```python
from build123d import *

# Parameters (mm, degrees)
FACE005_W        = 5
FACE005_H        = 52
EXTRUDE005_DEPTH = 1.6
FACE004_R        = 5
EXTRUDE004_DEPTH = 1.5
EXTRUDE003_DEPTH = 2
FACE002_R        = 1.25
EXTRUDE002_DEPTH = 10
FACE001_R        = 2.5
EXTRUDE001_DEPTH = 10
EXTRUDE_DEPTH    = 6.5


with BuildPart() as extrude005:
    # Face005 → Extrude005 (new body)
    with BuildSketch(Plane(origin=(34, 28, 5), x_dir=(0, 1, 0), z_dir=(0, 0, 1))):
        Rectangle(FACE005_W, FACE005_H)
    extrude(amount=-EXTRUDE005_DEPTH)


with BuildPart() as extrude004:
    # Face004 → Extrude004 (new body)
    with BuildSketch(Plane(origin=(34, 16.5, 6.5), x_dir=(0, 1, 0), z_dir=(0, 0, 1))):
        with BuildLine():
            ThreePointArc((15.5, 29), (14.328427, 31.828427), (11.5, 33))
            Line((11.5, 33), (-11.5, 33))
            ThreePointArc((-11.5, 33), (-14.328427, 31.828427), (-15.5, 29))
            Line((-15.5, 29), (-15.5, -29))
            ThreePointArc((-15.5, -29), (-14.328427, -31.828427), (-11.5, -33))
            Line((-11.5, -33), (11.5, -33))
            ThreePointArc((11.5, -33), (14.328427, -31.828427), (15.5, -29))
            Line((15.5, -29), (15.5, 29))
        make_face()
        with Locations((24.5, 26)):
            Circle(FACE004_R)
        with Locations((24.5, -26)):
            Circle(FACE004_R)
    extrude(amount=-EXTRUDE004_DEPTH)


with BuildPart() as extrude003:
    # Face003 → Extrude003 (new body)
    with BuildSketch(Plane(origin=(5, 5, 0), x_dir=(0, 1, 0), z_dir=(0, 0, 1))):
        Polygon((-1.443376, -2.5), (1.443376, -2.5), (2.886751, 0), (1.443376, 2.5), (-1.443376, 2.5), (-2.886751, 0), align=None)
        Polygon((24.443376, -60.5), (25.886751, -58), (24.443376, -55.5), (21.556624, -55.5), (20.113249, -58), (21.556624, -60.5), align=None)
        Polygon((1.443376, -60.5), (2.886751, -58), (1.443376, -55.5), (-1.443376, -55.5), (-2.886751, -58), (-1.443376, -60.5), align=None)
        Polygon((24.443376, -2.5), (25.886751, 0), (24.443376, 2.5), (21.556624, 2.5), (20.113249, 0), (21.556624, -2.5), align=None)
    extrude(amount=EXTRUDE003_DEPTH)


with BuildPart() as extrude002:
    # Face002 → Extrude002 (new body)
    with BuildSketch(Plane(origin=(63, 28, 6.5), x_dir=(0, 1, 0), z_dir=(0, 0, 1))):
        Circle(FACE002_R)
        with Locations((-23, 0)):
            Circle(FACE002_R)
        with Locations((-23, 58)):
            Circle(FACE002_R)
        with Locations((0, 58)):
            Circle(FACE002_R)
    extrude(amount=-EXTRUDE002_DEPTH)


with BuildPart() as extrude001:
    # Face001 → Extrude001 (new body)
    with BuildSketch(Plane(origin=(60, 41, 6.5), x_dir=(0, 1, 0), z_dir=(0, 0, 1))):
        Circle(FACE001_R)
        with Locations((0, 52)):
            Circle(FACE001_R)
    extrude(amount=-EXTRUDE001_DEPTH)


with BuildPart() as cut004:
    # Face → Extrude (new body)
    with BuildSketch(Plane(origin=(34, 24.5, 0), x_dir=(0, 1, 0), z_dir=(0, 0, 1))):
        with BuildLine():
            ThreePointArc((-19.5, 34), (-23.035534, 32.535534), (-24.5, 29))
            Line((-24.5, 29), (-24.5, -29.000001))
            ThreePointArc((-24.5, -29.000001), (-23.035534, -32.535534), (-19.5, -34))
            Line((-19.5, -34), (19.5, -34))
            ThreePointArc((19.5, -34), (23.035534, -32.535534), (24.5, -29))
            Line((24.5, -29), (24.5, 29))
            ThreePointArc((24.5, 29), (23.035534, 32.535534), (19.5, 34))
            Line((19.5, 34), (-19.5, 34))
        make_face()
    extrude(amount=EXTRUDE_DEPTH)

    # Cut: cut Extrude001
    add(extrude001.part, mode=Mode.SUBTRACT)

    # Cut001: cut Extrude002
    add(extrude002.part, mode=Mode.SUBTRACT)

    # Cut002: cut Extrude003
    add(extrude003.part, mode=Mode.SUBTRACT)

    # Cut003: cut Extrude004
    add(extrude004.part, mode=Mode.SUBTRACT)

    # Cut004: cut Extrude005
    add(extrude005.part, mode=Mode.SUBTRACT)


solid = cut004.part
```
Input: part model. Units: mm. Frame: model coordinates. A direction names the side the tool comes from. Give positions to 0.01 mm unless a question says otherwise; leave off trailing zeros. Loops run counter-clockwise (first coordinate to the right, second up) from the corner with the lowest first, then second, coordinate; pieces in that order, holes last. Notation, with made-up numbers: (38, -18.5) -> (81, -18.5) arc R6 cw to (81, -8.5) -> close; hole circle Ø4 at (-31.5, 89). An arc over 180 degrees is marked (long way). Use a Markdown table: item, result.
Q1. Section query A-A, the plane y = 41. Return the cut outline in (x, z).
Entries:
| item | result |
|---|---|
| outline | (0, 0) -> (5.5, 0) -> (5.5, 5) -> (3, 5) -> (3, 6.5) -> (0, 6.5) -> close; (10.5, 0) -> (57.5, 0) -> (57.5, 5) -> (55, 5) -> (55, 6.5) -> (13, 6.5) -> (13, 5) -> (10.5, 5) -> close; (62.5, 0) -> (68, 0) -> (68, 6.5) -> (65, 6.5) -> (65, 5) -> (62.5, 5) -> close |
Q2. Pull-direction query (Y, two-part tool) for faces 1 (the cylindrical face through (5.479, 29.155, 3.521)), 2 (the flat face through (67, 16, 6)), 3 (the flat face through (34, 24, 0)), 4 (the cylindrical face through (67, 47, 3)); classes: pulls with the +Y half, pulls with the -Y half, needs draft (parallel to the pull), parting line crosses it, or undercut.
Entries:
| item | result |
|---|---|
| face 1 | undercut |
| face 2 | undercut |
| face 3 | needs draft |
| face 4 | pulls with the +Y half |
Q3. Section query C-C, the plane x = 40. Return the cut outline in (y, z).
Entries:
| item | result |
|---|---|
| outline | (0, 0) -> (49, 0) -> (49, 6.5) -> (32, 6.5) -> (32, 5) -> (30.5, 5) -> (30.5, 3.4) -> (25.5, 3.4) -> (25.5, 5) -> (1, 5) -> (1, 6.5) -> (0, 6.5) -> close |
Q4. First-contact query: P1, Ø1.5, axis at x = 4, y = 5, coming from the -Z side; P2, Ø3, axis at x = 41, y = 9.5, coming from the +Z side. Flat tips, straight axial feed; report the tip coordinate or a pass-through.
Entries:
| item | result |
|---|---|
| P1 | stops at z = 2 |
| P2 | stops at z = 5 |
Q5. Section query B-B, the plane z = 1.25. State how many separate pieces and enclosed holes the cut face has, plus the area to 3 significant figures.
Entries:
| item | result |
|---|---|
| separate pieces | 1 |
| enclosed holes | 6 |
| area | 3,180 mm² |
Q6. Ray query, probe 1 along Y at (x, z) = (5, 3.4); probe 2 along X at (y, z) = (41, 1.4); probe 3 along Y at (x, z) = (60, 5.65). Return the intervals inside material, ascending. Write a range as from..to.
Entries:
| item | result |
|---|---|
| probe 1 | y = 0..3.75, 6.25..26.75, 29.25..49 |
| probe 2 | x = 0..5.5, 10.5..57.5, 62.5..68 |
| probe 3 | y = 0..1, 32..36, 46..49 |
Q7. Access query for faces 5 (the flat face through (34, 0, 3)), 6 (the flat face through (3.768, 30.175, 0.986)), 7 (the flat face through (34, 30.5, 4)). Directions: +Z, -Z, +X, -X, +Y, -Y. A direction counts if a zero-diameter tool reaches every point of the face in a straight line with its end or side. Return the directions, or none.
Entries:
| item | result |
|---|---|
| face 5 | +Z, -Z, +X, -X, -Y |
| face 6 | -Z |
| face 7 | +Z |
